Here's how the part is built. I have some questions about the finished solid (model axes, mm). A direction names the side the tool comes from. Coordinates: 2 decimals unless noted, no trailing zeros. Loops run counter-clockwise (first coordinate to the right, second up) from the corner with the lowest first, then second, coordinate; pieces in that order, holes last. Notation, with made-up numbers: M -2,16 L 34,16 A29 cw 34,49 Z; hole C 43.25,-7 d8. An arc over 180 degrees is marked long. Use one line per item in the form item = value. Start each with the question number.
(1) Imagine slicing it at A-A, the plane z = 0. Please give me the cut outline in (x, y) (3 decimals), and give its area (3 significant figures).
(2) Imagine slicing it at C-C, the plane y = 0. State how many separate pieces and enclosed holes the cut face has, and give its area (3 significant figures).
(3) Please list where these lines run through material, in increasing order: L1, parallel to X at y = 0, z = 1.25; L2, parallel to Z at x = 10, y = 0 (3 decimals).
(4) Will these pins go through, and if not, where does the flat tip stop? P1, Ø3, axis at x = 19, y = -1.5, coming from the +Z side; P2, Ø5, axis at x = 22.5, z = -2, coming from the -Y side; P3, Ø6, axis at x = 10, z = 0, coming from the -Y side.
(5) Thinking about a two-plate mould opening in X: for faces 4 (the flat face through (9.268, -3, -1)), 5 (the cylindrical face through (19.212, 0.766, 1.847)), 6 (the cylindrical face through (12.675, 0.688, 0.358)), which applies, +X half, -X half, draft (parallel to the pull), parting line (faces both ways), or undercut?
(6) On a 3-axis mill with a long thin cutter (end or side, diameter ignored), from which of +Z, -Z, +X, -X, +Y, -Y can I reach the whole of each face in a straight line? I mean faces 1 (the cylindrical face through (2.86, -1.5, 4.77)), 2 (the flat face through (25, 1, -1)), 3 (the flat face through (15.268, 2, -1)). Say none if no direction works.
(7) Imagine slicing it at B-B, the plane x = 12.25. Please give me the cut outline in (y, z) (3 decimals).
```python
from build123d import *

# Parameters (mm, degrees)
F2_R     = 0.5
F3_DEPTH = 12.5


with BuildPart() as f1:
    # F0 (on Front) → F1 (revolve)
    with BuildSketch(Plane.XZ):
        Polygon((1, 5), (0, 6), (0, 0.775), (25, 0.775), (25, 3), (23.267949, 2), (15.267949, 2), (15.267949, 3), (9.267949, 3), (9.267949, 4), (4.767949, 4), (4.767949, 5), align=None)
    revolve(axis=Axis((6.044726, 0, 0), (1, 0, 0)))

    # F2 (on Top) → F3 (cut, symmetric)
    with BuildSketch(Plane.XY):
        with Locations((3.057949, 0)):
            Circle(F2_R)
        with Locations((8.358715, 0)):
            Circle(F2_R)
        with Locations((13.456892, 0)):
            Circle(F2_R)
        with Locations((22.136655, 0)):
            Circle(F2_R)
    extrude(amount=F3_DEPTH, both=True, mode=Mode.SUBTRACT)


solid = f1.part
```
Answer:
q1.outline = M 0,-6 L 1,-5 L 4.768,-5 L 4.768,-4 L 9.268,-4 L 9.268,-3 L 15.268,-3 L 15.268,-2 L 23.268,-2 L 25,-3 L 25,-0.775 L 0,-0.775 Z; M 0,0.775 L 25,0.775 L 25,3 L 23.268,2 L 15.268,2 L 15.268,3 L 9.268,3 L 9.268,4 L 4.768,4 L 4.768,5 L 1,5 L 0,6 Z
q1.area = 123 mm²
q2.separate_pieces = 10
q2.enclosed_holes = 0
q2.area = 101 mm²
q3.L1 = 0 to 2.56, 3.56 to 7.86, 8.86 to 12.96, 13.96 to 21.64, 22.64 to 25
q3.L2 = -3 to -0.775, 0.775 to 3
q4.P1 = 2
q4.P2 = -2.71
q4.P3 = -4
q5.face_4 = +X half
q5.face_5 = undercut
q5.face_6 = draft
q6.face_1 = +X
q6.face_2 = +Z, -Z, +X, +Y, -Y
q6.face_3 = none
q7.outline = C 0,0 d6; hole C 0,0 d1.55
